from build123d import *

# Parameters (mm, degrees)
F1_DEPTH = 12
F2_R     = 1.25
F3_DEPTH = 25


with BuildPart() as f1:
    # F0 (on Top) → F1 (new body)
    with BuildSketch(Plane.XY):
        Polygon((-8.13678, -6.502725), (-6.13678, -6.502725), (-6.13678, -1.002725), (-6.13678, 5.497275), (-3.23678, 5.497275), (-3.23678, -6.502725), (-1.23678, -6.502725), (-1.23678, 7.497275), (-8.13678, 7.497275), align=None)
        Polygon((-6.13678, -1.002725), (-6.13678, -6.502725), (-5.13678, -5.295739), (-5.13678, -1.002725), align=None)
    extrude(amount=F1_DEPTH)

    # F2 (on face) → F3 (cut)
    with BuildSketch(Plane(origin=(-8.13678, 0, 0), x_dir=(0, -1, 0), z_dir=(-1, 0, 0))):
        with Locations((3.502725, 6)):
            Circle(F2_R)
    extrude(amount=-F3_DEPTH, mode=Mode.SUBTRACT)


solid = f1.part
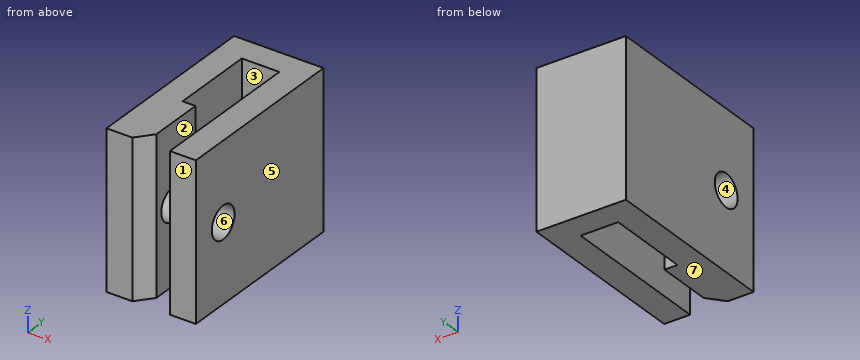
Could you check a few things on this model? Use its own coordinates, in mm. Face numbers are marked on the shaded views. A direction names the side the tool comes from. Coordinates: 2 decimals unless noted, no trailing zeros. Loops run counter-clockwise (first coordinate to the right, second up) from the corner with the lowest first, then second, coordinate; pieces in that order, holes last.
1. I need wall thicknesses on L1, parallel to X at y = -4.75, z = 5; L2, parallel to X at y = 3, z = 5.75; L3, parallel to Y at x = -5.5, z = 6.5. Which ranges of each line are inside material? Lowest first, please.
2. Imagine slicing it at D-D (z = 1.25). Please give me the cut outline in (x, y), and give its area (3 significant figures).
3. For the marked faces 1, 2 and 3, which set-ups out of +Z, -Z, +X, -X, +Y, -Y let a thin tool reach every point of the face, with its end or its side?
4. We'd pull the mould along Z, two halves only. Please class the marked faces 4, 5, 6 and 7: released by +Z, released by -Z, zero draft, split by the parting line, or undercut.
5. Imagine slicing it at B-B (x = -5.75). Please give me the cut outline in (y, z).
6. For P1, Ø2, axis at y = -3.5, z = 6, coming from the +X side, with a flat end and sliding along its axis, tell me the tip position at first contact or that it passes through.
7. Imagine slicing it at C-C (z = 6). Please give me the cut outline in (x, y).
8. Imagine slicing it at A-A (y = 2.25). Please give me the cut outline in (x, z), and give its area (3 significant figures).
Computed values:
1. L1: x = -8.14 to -5.14, -3.24 to -1.24
1. L2: x = -8.14 to -6.14, -3.24 to -1.24
1. L3: y = -5.73 to -4.65, -2.36 to -1, 5.5 to 7.5
2. outline: (-8.14, -6.5) - (-6.14, -6.5) - (-5.14, -5.3) - (-5.14, -1) - (-6.14, -1) - (-6.14, 5.5) - (-3.24, 5.5) - (-3.24, -6.5) - (-1.24, -6.5) - (-1.24, 7.5) - (-8.14, 7.5) - close
2. area: 66.7 mm2
3. face 1: +Z, -Z, +X, -X, -Y
3. face 2: +Z, -Z, -Y
3. face 3: +Z, -Z
4. face 4: undercut
4. face 5: zero draft
4. face 6: undercut
4. face 7: released by -Z
5. outline: (-6.04, 0) - (-1, 0) - (-1, 12) - (-6.04, 12) - close; (5.5, 0) - (7.5, 0) - (7.5, 12) - (5.5, 12) - close; hole circle Ø2.5 at (-3.5, 6)
6. P1: passes through
7. outline: (-8.14, -6.5) - (-6.14, -6.5) - (-5.14, -5.3) - (-5.14, -4.75) - (-8.14, -4.75) - close; (-8.14, -2.25) - (-5.14, -2.25) - (-5.14, -1) - (-6.14, -1) - (-6.14, 5.5) - (-3.24, 5.5) - (-3.24, -2.25) - (-1.24, -2.25) - (-1.24, 7.5) - (-8.14, 7.5) - close; (-3.24, -6.5) - (-1.24, -6.5) - (-1.24, -4.75) - (-3.24, -4.75) - close
8. outline: (-8.14, 0) - (-6.14, 0) - (-6.14, 12) - (-8.14, 12) - close; (-3.24, 0) - (-1.24, 0) - (-1.24, 12) - (-3.24, 12) - close
8. area: 48.0 mm2
